Model file for the job. Use its own axes, mm. A direction names the side the tool comes from. Coordinates: 2 decimals unless noted, no trailing zeros. Write each loop counter-clockwise with the first axis right and the second up, starting at its lowest first coordinate (ties: lowest second). Pieces come first, ordered by that corner, then holes. Notation, with made-up numbers: M 54,60 L 88,60 A23 ccw 88,85 Z; hole C 11.5,-7.5 d7. An arc over 180 degrees is marked long. Put each result on its own line as item: value. Start each with the question number.
Q1. Pull direction Z, two halves, no side cores. Call faces 3 (the flat face through (563, 25, -50.8)), 4 (the flat face through (563, 25, -46.037)), 5 (the flat face through (563, 25, 0)), 6 (the flat face through (563, 0, -25)): pulls with the +Z half, pulls with the -Z half, needs draft (parallel to the pull), parting line crosses it, or undercut.
Q2. Drill centre lines: line 1 along Z through (x, y) = (304.8, 2.65); line 2 along Y through (x, z) = (663, -11); line 3 along Z through (x, y) = (1010.5, 31.5). Where is each one in solid material? Low to high.
Q3. Which spindle directions (+Z, -Z, +X, -X, +Y, -Y) get a long thin tool onto all of the face, cutting with end or side? Do faces 1 (the flat face through (563, 4.762, -25)), 2 (the flat face through (563, 50.8, -25)). Say none if no direction does.
Q4. Drop flat-ended pins along their axis: pin 1 (4 mm diameter, centred on x = 25.4, y = 25.4, fed in from -Z) (1 decimal); pin 2 (4 mm diameter, centred on x = 304.8, z = -25.4, fed in from -Y). Give the stop position or say it passes through.
Q5. Cut at A-A (x = 985.5). Write the cut outline in (y, z), then the cut area to 3 significant figures.
Q6. Cut at B-B (z = -37.5). Write the cut outline in (x, y), then the cut area to 3 significant figures.
```python
from build123d import *

# Parameters (mm, degrees)
SKETCH1_W           = 50.8
SKETCH1_H           = 50.8
SKETCH1_W_2         = 41.275
SKETCH1_H_2         = 41.275
BOSS_EXTRUDE1_DEPTH = 1143
SKETCH2_R           = 2.38125
CUT_EXTRUDE1_DEPTH  = 51.8
LPATTERN1_COUNT     = 6
LPATTERN1_PITCH     = 203.2
SKETCH3_R           = 2.38125
CUT_EXTRUDE2_DEPTH  = 4.7625
LPATTERN2_COUNT     = 6
LPATTERN2_PITCH     = 203.2


with BuildPart() as part:
    # Sketch1 → Boss-Extrude1 (new body)
    with BuildSketch(Plane(origin=(0, 0, 0), x_dir=(0, 0, -1), z_dir=(1, 0, 0))):
        with Locations((25.4, 25.4)):
            Rectangle(SKETCH1_W, SKETCH1_H)
        with Locations((25.4, 25.4)):
            Rectangle(SKETCH1_W_2, SKETCH1_H_2, mode=Mode.SUBTRACT)
    extrude(amount=BOSS_EXTRUDE1_DEPTH)

    # Sketch2 → Cut-Extrude1 (cut, through all)
    with BuildSketch(Plane(origin=(0, 0, -50.8), x_dir=(-1, 0, 0), z_dir=(0, 0, -1))):
        with Locations((-1041.4, 25.4)):
            Circle(SKETCH2_R)
    cut_extrude1 = extrude(amount=-CUT_EXTRUDE1_DEPTH, mode=Mode.SUBTRACT)

    # LPattern1: Cut-Extrude1 ×6
    with Locations(*[(-i * LPATTERN1_PITCH, 0, 0) for i in range(1, LPATTERN1_COUNT)]):
        add(cut_extrude1, mode=Mode.SUBTRACT)

    # Sketch3 → Cut-Extrude2 (cut)
    with BuildSketch(Plane.XZ):
        with Locations((101.6, -25.4)):
            Circle(SKETCH3_R)
    cut_extrude2 = extrude(amount=-CUT_EXTRUDE2_DEPTH, mode=Mode.SUBTRACT)

    # LPattern2: Cut-Extrude2 ×6
    with Locations(*[(i * LPATTERN2_PITCH, 0, 0) for i in range(1, LPATTERN2_COUNT)]):
        add(cut_extrude2, mode=Mode.SUBTRACT)


solid = part.part
```
Computed values:
1. face 3: pulls with the -Z half
1. face 4: undercut
1. face 5: pulls with the +Z half
1. face 6: needs draft
2. line 1: -50.8 to -27.78, -23.02 to 0
2. line 2: 0 to 4.76, 46.04 to 50.8
2. line 3: -50.8 to -46.04, -4.76 to 0
3. face 1: +X, -X
3. face 2: +Z, -Z, +X, -X, +Y
4. pin 1: through
4. pin 2: y = 46.04
5. outline: M 0,-50.8 L 50.8,-50.8 L 50.8,0 L 0,0 Z; hole M 4.76,-46.04 L 46.04,-46.04 L 46.04,-4.76 L 4.76,-4.76 Z
5. area: 877 mm2
6. outline: M 0,0 L 1143,0 L 1143,4.76 L 0,4.76 Z; M 0,46.04 L 1143,46.04 L 1143,50.8 L 0,50.8 Z
6. area: 10,900 mm2
